CAD build for the part. Positions are in the model's coordinates, mm. A direction names the side the tool comes from. Give positions to 0.01 mm unless a question says otherwise; leave off trailing zeros. Loops run counter-clockwise (first coordinate to the right, second up) from the corner with the lowest first, then second, coordinate; pieces in that order, holes last. Notation, with made-up numbers: M 10.25,-1.75 L 69.25,-1.75 A31 cw 69.25,36.25 Z; hole C 55.5,-3 d6. An arc over 180 degrees is marked long. Answer as CSV lines item,"result".
Autodesk Inventor part; units mm, degrees
ref_plane "YZ Plane" through (0, 0, 0) normal (1, 0, 0) x (0, 1, 0)
ref_plane "XZ Plane" through (0, 0, 0) normal (0, 1, 0) x (-1, 0, 0)
ref_plane "XY Plane" through (0, 0, 0) normal (0, 0, 1) x (1, 0, 0)
sketch "Sketch1" plane through (0, 0, 0) normal (0, 0, 1) x (1, 0, 0)
  line L0 (-4, 5) -> (4, 5)
  line L1 (4, 5) -> (4, -5)
  line L2 (4, -5) -> (-4, -5)
  line L3 (-4, -5) -> (-4, 5)
  line L4 (-4, 5) -> (4, -5) construction
  line L5 (4, 5) -> (-4, -5) construction
  point P0 (0, 0)
  dimension "d0" = 8
  dimension "d1" = 10
extrude "Extrusion1" add sketch "Sketch1" along normal blind 1.5
sketch "Sketch2" plane through (0, 0, 1.5) normal (0, 0, 1) x (1, 0, 0)
  line L0 (-4, -5) -> (4, -5)
  line L1 (4, -5) -> (4, 5)
  line L2 (4, 5) -> (-4, 5)
  line L3 (-4, 5) -> (-4, -5)
  line L4 (-5.6, 0) -> (5.6, 0)
  line L5 (0, -7) -> (0, 7)
  line L6 (4, 5) -> (-4, 5)
  line L7 (-2.25, 5) -> (2.25, 5)
  line L8 (2.25, 5) -> (2.25, -2)
  line L9 (2.25, -2) -> (-2.25, -2)
  line L10 (-2.25, -2) -> (-2.25, 5)
  point P0 (0, 0)
  dimension "d4" = 4.5
  dimension "d5" = 7
extrude "Extrusion2" cut sketch "Sketch2" against normal through all contours L9 L10 L4 L5 | L5 L4 L8 L9 | L10 L2 L5 L4 | L5 L2 L8 L4
fillet "Fillet1" radius 0.4 4 edges at (-4, 0, 1.5) (-4, 0, 0) (4, 0, 0) (4, 0, 1.5)
equation "\"BendRadius\" = Thickness"
equation "\"BendReliefWidth\" = Thickness"
equation "\"BendReliefDepth\" = 0.5 * Thickness"
equation "\"CornerReliefSize\" = 4 * Thickness"
equation "\"MinimumRemnant\" = 2 * Thickness"
equation "\"TransitionRadius\" = BendRadius"
equation "\"JacobiRadiusSize\" = BendRadius"
equation "\"GapSize\" = Thickness"
properties part number "_3DPrint"
Q1. Cut at B-B (z = 0.6). Write the cut outline in (x, y).
Solution:
outline,"M -4,-5 L 4,-5 L 4,5 L 2.25,5 L 2.25,-2 L -2.25,-2 L -2.25,5 L -4,5 Z"
Q2. Which spindle directions (+Z, -Z, +X, -X, +Y, -Y) get a long thin tool onto all of the face, cutting with end or side? Do faces 1 (the flat face through (0, -5, 1)), 2 (the flat face through (0, -2, 1)). Say none if no direction does.
Solution:
face 1,"+Z, -Z, +X, -X, -Y"
face 2,"+Z, -Z, +Y"
Q3. Mould opens along X. For faces 3 (the flat face through (2.25, 2, 1)), 4 (the flat face through (-0.1, -2.2, 1.5)), 5 (the flat face through (-2.25, 1, 1)) say: released by +X, released by -X, zero draft, split by the parting line, or undercut.
Solution:
face 3,"undercut"
face 4,"zero draft"
face 5,"undercut"
Q4. Cut at A-A (y = 1.5). Write the cut outline in (x, z).
Solution:
outline,"M -4,0.4 A0.4 ccw -3.6,0 L -2.25,0 L -2.25,1.5 L -3.6,1.5 A0.4 ccw -4,1.1 Z; M 2.25,0 L 3.6,0 A0.4 ccw 4,0.4 L 4,1.1 A0.4 ccw 3.6,1.5 L 2.25,1.5 Z"
Q5. Cut at C-C (x = 1). Write the cut outline in (y, z), and give its area (3 significant figures).
Solution:
outline,"M -5,0 L -2,0 L -2,1.5 L -5,1.5 Z"
area,"4.50 mm²"
Q6. Wall check: line 1 (X direction, y = -1.25, z = 0.75); line 2 (Y direction, x = 0.25, z = 0.35); line 3 (X direction, y = 3, z = 0.15). Give the ranges that are in metal, low to high. Write a range as [from, to].
Solution:
line 1,"x = [-4, -2.25], [2.25, 4]"
line 2,"y = [-5, -2]"
line 3,"x = [-3.91, -2.25], [2.25, 3.91]"
